Design review of the part built by this model. Coordinates are the model's own, in mm. Face numbers are marked on the shaded views. A direction names the side the tool comes from. Coordinates: 2 decimals unless noted, no trailing zeros. Write each loop counter-clockwise with the first axis right and the second up, starting at its lowest first coordinate (ties: lowest second). Pieces come first, ordered by that corner, then holes. Notation, with made-up numbers: (-16.5, 16.25) - (-12.5, 16.25) arc R31 cw to (-12.5, 40.25) - close; hole circle Ø1 at (74.5, 38). An arc over 180 degrees is marked (long way). One line per item, written item: value.
from build123d import *

# Parameters (mm, degrees)
CUT_EXTRUDE1_DEPTH = 2.08
FILLET1_R          = 0.25
CHAMFER1_SIZE      = 0.625


with BuildPart() as part:
    # Sketch1 → Revolve1 (revolve)
    with BuildSketch(Plane.XY, mode=Mode.PRIVATE) as revolve1_sk:
        with BuildLine():
            Line((0, 0), (2.85, 0))
            ThreePointArc((2.85, 0), (4.547056275, -0.702943725), (5.25, -2.4))
            Line((5.25, -2.4), (5.25, -3.2))
            Line((5.25, -3.2), (3, -3.2))
            Line((3, -3.2), (3, -19.2))
            Line((3, -19.2), (0, -19.2))
            Line((0, -19.2), (0, 0))
        make_face()
    revolve(revolve1_sk.sketch.rotate(Axis((0, 5, 0), (0, -1, 0)), 180), axis=Axis((0, 5, 0), (0, -1, 0)))

    # Sketch2 → Cut-Extrude1 (cut)
    with BuildSketch(Plane(origin=(0, 0, 0), x_dir=(1, 0, 0), z_dir=(0, 1, 0))):
        Polygon((2.309401077, 0), (1.154700538, 2), (-1.154700538, 2), (-2.309401077, 0), (-1.154700538, -2), (1.154700538, -2), align=None)
    extrude(amount=-CUT_EXTRUDE1_DEPTH, mode=Mode.SUBTRACT)

    # Fillet1
    fillet1_edges = [part.edges().sort_by_distance(p)[0] for p in [
        (3, -3.2, 0),
    ]]
    fillet(fillet1_edges, radius=FILLET1_R)

    # Chamfer1
    chamfer1_edges = [part.edges().sort_by_distance(p)[0] for p in [
        (3, -19.2, 0),
    ]]
    chamfer(chamfer1_edges, length=CHAMFER1_SIZE)


solid = part.part
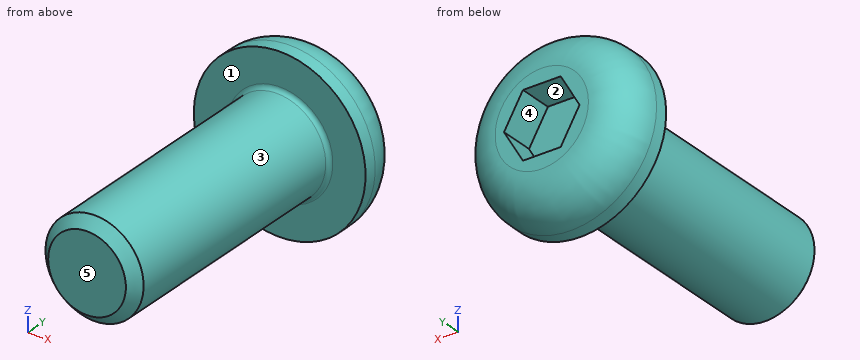
1. Consider section B-B, the plane y = -11.5. Write out the cut boundary in (x, z), then the cut area to 3 significant figures.
Answer block:
outline: circle Ø6 at (0, 0)
area: 28.3 mm^2
2. Insertion check: pin 1 Ø3 at (x, z) = (1, 0) entering from +Y; pin 2 Ø1 at (x, y) = (0.5, -1.5) entering from -Z; pin 3 Ø1 at (y, z) = (-15, 0) entering from +X; pin 4 Ø6 at (x, y) = (-2, -11) entering from -Z. Each pin has a flat end and moves straight along its axis. Give the tip position at first contact, or say it passes through.
Answer block:
pin 1: stops at y = 0
pin 2: stops at z = -5.2
pin 3: stops at x = 3
pin 4: stops at z = -3
3. Mouldability with a two-part tool opening along X and no side actions: class the marked faces 1, 2 and 3 as released by +X, released by -X, zero draft, split by the parting line, or undercut.
Answer block:
face 1: zero draft
face 2: undercut
face 3: split by the parting line
4. For the marked faces 4 and 5, list the 3-axis set-ups (+Z, -Z, +X, -X, +Y, -Y) from which the entire face can be reached by the end or side of a thin tool; tool diameter is ignored.
Answer block:
face 4: +Y
face 5: +Z, -Z, +X, -X, -Y
5. Consider section A-A, the plane x = 0. Write out the cut boundary in (y, z) (3 decimals), then the cut area to 3 significant figures.
Answer block:
outline: (-19.2, -2.375) - (-18.575, -3) - (-3.45, -3) arc R0.25 cw to (-3.2, -3.25) - (-3.2, -5.25) - (-2.4, -5.25) arc R2.4 ccw to (0, -2.85) - (0, -2) - (-2.08, -2) - (-2.08, 2) - (0, 2) - (0, 2.85) arc R2.4 ccw to (-2.4, 5.25) - (-3.2, 5.25) - (-3.2, 3.25) arc R0.25 cw to (-3.45, 3) - (-18.575, 3) - (-19.2, 2.375) - close
area: 118 mm^2
6. Wall thickness on line 1 along Y through (x, z) = (-0.5, -0.75); line 2 along Y through (x, z) = (2.5, -1.25); line 3 along X through (y, z) = (-14.75, 0.25): over which ranges is each line inside the solid? List them lowest first.
Answer block:
line 1: y = -19.2 to -2.08
line 2: y = -18.78 to 0
line 3: x = -2.99 to 2.99
